Read the model definition and answer for the solid it produces. Units are mm, in the model's axes. A direction names the side the tool comes from. Round coordinates to 2 decimals unless told otherwise and drop trailing zeros. Write each loop counter-clockwise with the first axis right and the second up, starting at its lowest first coordinate (ties: lowest second). Pieces come first, ordered by that corner, then holes.
from build123d import *

# Parameters (mm, degrees)
CROQUIS1_W                = 7
CROQUIS1_H                = 18
SALIENTE_EXTRUIR1_DEPTH   = 9
SALIENTE_EXTRUIR1_2_DEPTH = 9
SALIENTE_EXTRUIR1_3_DEPTH = 9
SALIENTE_EXTRUIR1_4_DEPTH = 9
CROQUIS2_W                = 24.75
CROQUIS2_H                = 4
SALIENTE_EXTRUIR2_DEPTH   = 9
CROQUIS3_R                = 2.5
CROQUIS3_R_2              = 2
SALIENTE_EXTRUIR3_DEPTH   = 5.5
CROQUIS4_R                = 1
CORTAR_EXTRUIR1_DEPTH     = 38.59072359
CROQUIS5_W                = 6
CROQUIS5_H                = 8
CORTAR_EXTRUIR2_DEPTH     = 40.272286666


with BuildPart() as part:
    # Croquis1 → Saliente-Extruir1 (new body)
    with BuildSketch(Plane.XY):
        with Locations((11.75, 9)):
            Rectangle(CROQUIS1_W, CROQUIS1_H)
    extrude(amount=SALIENTE_EXTRUIR1_DEPTH)



with BuildPart() as body_2:
    # Croquis1 → Saliente-Extruir1 2 (new body)
    with BuildSketch(Plane.XY):
        with Locations((3.5, 9)):
            Rectangle(CROQUIS1_W, CROQUIS1_H)
    extrude(amount=SALIENTE_EXTRUIR1_2_DEPTH)


with BuildPart() as body_3:
    # Croquis1 → Saliente-Extruir1 3 (new body)
    with BuildSketch(Plane.XY):
        with Locations((20, 9)):
            Rectangle(CROQUIS1_W, CROQUIS1_H)
    extrude(amount=SALIENTE_EXTRUIR1_3_DEPTH)


with BuildPart() as body_4:
    # Croquis1 → Saliente-Extruir1 4 (new body)
    with BuildSketch(Plane.XY):
        with Locations((28.25, 9)):
            Rectangle(CROQUIS1_W, CROQUIS1_H)
    extrude(amount=SALIENTE_EXTRUIR1_4_DEPTH)


with BuildPart() as part_1:
    add(part.part)

    add(body_2.part)  # Saliente-Extruir2 merges body 2

    add(body_3.part)  # Saliente-Extruir2 merges body 3

    add(body_4.part)  # Saliente-Extruir2 merges body 4
    # Croquis2 → Saliente-Extruir2 (add)
    with BuildSketch(Plane.XY):
        with Locations((12.375, 9)):
            Rectangle(CROQUIS2_W, CROQUIS2_H)
    extrude(amount=SALIENTE_EXTRUIR2_DEPTH)

    # Croquis3 → Saliente-Extruir3 (add)
    # profile 1 of 8: a face of its own
    with BuildSketch(Plane.XY.offset(9)):
        with Locations(Location((3.5, 12, 0), (0, 0, 180))):
            Circle(CROQUIS3_R)
        with Locations((3.5, 12)):
            Circle(CROQUIS3_R_2, mode=Mode.SUBTRACT)
    # profile 2 of 8: a face of its own
    with BuildSketch(Plane.XY.offset(9)):
        with Locations(Location((11.75, 12, 0), (0, 0, 180))):
            Circle(CROQUIS3_R)
        with Locations((11.75, 12)):
            Circle(CROQUIS3_R_2, mode=Mode.SUBTRACT)
    # profile 3 of 8: a face of its own
    with BuildSketch(Plane.XY.offset(9)):
        with Locations(Location((20, 12, 0), (0, 0, 180))):
            Circle(CROQUIS3_R)
        with Locations((20, 12)):
            Circle(CROQUIS3_R_2, mode=Mode.SUBTRACT)
    # profile 4 of 8: a face of its own
    with BuildSketch(Plane.XY.offset(9)):
        with Locations(Location((28.25, 12, 0), (0, 0, 180))):
            Circle(CROQUIS3_R)
        with Locations((28.25, 12)):
            Circle(CROQUIS3_R_2, mode=Mode.SUBTRACT)
    # profile 5 of 8: a face of its own
    with BuildSketch(Plane.XY.offset(9)):
        with Locations(Location((11.75, 6, 0), (0, 0, 180))):
            Circle(CROQUIS3_R)
        with Locations((11.75, 6)):
            Circle(CROQUIS3_R_2, mode=Mode.SUBTRACT)
    # profile 6 of 8: a face of its own
    with BuildSketch(Plane.XY.offset(9)):
        with Locations(Location((20, 6, 0), (0, 0, 180))):
            Circle(CROQUIS3_R)
        with Locations((20, 6)):
            Circle(CROQUIS3_R_2, mode=Mode.SUBTRACT)
    # profile 7 of 8: a face of its own
    with BuildSketch(Plane.XY.offset(9)):
        with Locations(Location((28.25, 6, 0), (0, 0, 180))):
            Circle(CROQUIS3_R)
        with Locations((28.25, 6)):
            Circle(CROQUIS3_R_2, mode=Mode.SUBTRACT)
    # profile 8 of 8: a face of its own
    with BuildSketch(Plane.XY.offset(9)):
        with Locations(Location((3.5, 6, 0), (0, 0, 180))):
            Circle(CROQUIS3_R)
        with Locations((3.5, 6)):
            Circle(CROQUIS3_R_2, mode=Mode.SUBTRACT)
    extrude(amount=SALIENTE_EXTRUIR3_DEPTH)

    # Croquis4 → Cortar-Extruir1 (cut, through all)
    with BuildSketch(Plane.XY.offset(9)):
        with Locations((7.625, 9)):
            Circle(CROQUIS4_R)
        with Locations((15.875, 9)):
            Circle(CROQUIS4_R)
        with Locations((24.125, 9)):
            Circle(CROQUIS4_R)
    extrude(amount=-CORTAR_EXTRUIR1_DEPTH, mode=Mode.SUBTRACT)

    # Croquis5 → Cortar-Extruir2 (cut, through all)
    with BuildSketch(Plane.XZ):
        with Locations((3.5, 4.5)):
            Rectangle(CROQUIS5_W, CROQUIS5_H)
        with Locations((11.75, 4.5)):
            Rectangle(CROQUIS5_W, CROQUIS5_H)
        with Locations((20, 4.5)):
            Rectangle(CROQUIS5_W, CROQUIS5_H)
        with Locations((28.25, 4.5)):
            Rectangle(CROQUIS5_W, CROQUIS5_H)
    extrude(amount=-CORTAR_EXTRUIR2_DEPTH, mode=Mode.SUBTRACT)


solid = part_1.part
Q1. Flat-ended cylindrical pins translate along their axes: pin 1 Ø0.6 at (x, z) = (24, 3.5) entering from +Y; pin 2 Ø2 at (x, y) = (20, 6) entering from +Z. Find the tip coordinate at first contact, or state that the pin passes through.
Verdict:
pin 1: stops at y = 11
pin 2: stops at z = 9
Q2. Straight lines are drawn through the part: probe 1 along Y at (x, z) = (3.5, 13.1); probe 2 along Z at (x, y) = (10.5, 11); probe 3 along Z at (x, y) = (10, 4.25). For each, find the intervals that lie inside material, in ascending order.
Verdict:
probe 1: y = 3.5 to 4, 8 to 8.5, 9.5 to 10, 14 to 14.5
probe 2: z = 0 to 0.5, 8.5 to 9
probe 3: z = 0 to 0.5, 8.5 to 14.5
Q3. Determine the mould class of faces 6 (the flat face through (14, 6, 14.5)), 7 (the flat face through (16.5, 3, 4)) for opening direction X: pulls with the +X half, pulls with the -X half, needs draft (parallel to the pull), parting line crosses it, or undercut.
Verdict:
face 6: needs draft
face 7: undercut
Q4. Section A-A (x = 20) is taken. Determine the outline of the cut face in (y, z).
Verdict:
outline: (0, 0) - (18, 0) - (18, 0.5) - (0, 0.5) - close; (0, 8.5) - (18, 8.5) - (18, 9) - (14.5, 9) - (14.5, 14.5) - (14, 14.5) - (14, 9) - (10, 9) - (10, 14.5) - (9.5, 14.5) - (9.5, 9) - (8.5, 9) - (8.5, 14.5) - (8, 14.5) - (8, 9) - (4, 9) - (4, 14.5) - (3.5, 14.5) - (3.5, 9) - (0, 9) - close
Q5. Which of the six approach directions +Z, -Z, +X, -X, +Y, -Y give full straight-line access (tool end or side, diameter ignored) to faces 1 (the flat face through (7, 3, 4)), 2 (the flat face through (0.5, 9, 4)), 3 (the flat face through (16, 11, 4)), 4 (the cylindrical face through (30.234, 13.521, 11.712)), 5 (the flat face through (19, 9, 0))?
Verdict:
face 1: +Z, -Z, -Y
face 2: +Y, -Y
face 3: +Z, -Z, +Y
face 4: +Z
face 5: -Z, +X, -X, +Y, -Y
Q6. Section B-B (y = 9) is taken. State how many separate pieces and enclosed holes the cut face has, then the cut area to 4 significant figures.
Verdict:
separate pieces: 4
enclosed holes: 4
area: 39.75 mm2
